```python
from build123d import *

# Parameters (mm, degrees)
F0_R     = 110
F0_R_2   = 1.75
F1_DEPTH = 3


with BuildPart() as f1:
    # F0 (on Top) → F1 (new body)
    with BuildSketch(Plane.XY):
        Circle(F0_R)
        with Locations((-91.582186, -52.875)):
            Circle(F0_R_2, mode=Mode.SUBTRACT)
        with Locations((0, -105.75)):
            Circle(F0_R_2, mode=Mode.SUBTRACT)
        with Locations((91.582186, -52.875)):
            Circle(F0_R_2, mode=Mode.SUBTRACT)
        with Locations((-91.582186, 52.875)):
            Circle(F0_R_2, mode=Mode.SUBTRACT)
        with Locations((91.582186, 52.875)):
            Circle(F0_R_2, mode=Mode.SUBTRACT)
        with Locations((0, 105.75)):
            Circle(F0_R_2, mode=Mode.SUBTRACT)
    extrude(amount=F1_DEPTH)


solid = f1.part
```
Here's how the part is built. I have some questions about the finished solid (model axes, mm). Give positions to 0.01 mm unless a question says otherwise; leave off trailing zeros. Loops run counter-clockwise (first coordinate to the right, second up) from the corner with the lowest first, then second, coordinate; pieces in that order, holes last. Notation, with made-up numbers: M 5.5,46 L 55.5,46 A17 cw 55.5,66 Z; hole C 25,-25.75 d1. An arc over 180 degrees is marked long. Use one line per item in the form item = value. Start each with the question number.
Q1. Thinking about a two-plate mould opening in Y: for faces 1 (the flat face through (-2, 2, 3)), 2 (the cylindrical face through (-23.846, -107.384, 1.479)), which applies, +Y half, -Y half, draft (parallel to the pull), parting line (faces both ways), or undercut?
Q2. Will these pins go through, and if not, where does the flat tip stop? pin 1 Ø1 at (y, z) = (-42.5, 2) entering from -X; pin 2 Ø5 at (x, y) = (-69, -82) entering from -Z; pin 3 Ø1.5 at (x, z) = (81, 2) entering from -Y.
Q3. If we section it at B-B (y = -73): Write out the boundary of the cut face in (x, z).
Q4. If we section it at A-A (z = 1.7): Write out the boundary of the cut face in (x, y) (3 decimals), then the cut area to 3 significant figures.
Q5. If we section it at C-C (x = -29.5): Write out the boundary of the cut face in (y, z).
Q6. I need wall thicknesses on line 1 along Y through (x, z) = (0, 1.9); line 2 along Y through (x, z) = (-90, 1.9); line 3 along Y through (x, z) = (14, 0.2). Which ranges of each line are inside material? Lowest first, please.
Taken from the geometry:
q1.face_1 = draft
q1.face_2 = parting line
q2.pin_1 = -101.67
q2.pin_2 = 0
q2.pin_3 = -75.23
q3.outline = M -82.29,0 L 82.29,0 L 82.29,3 L -82.29,3 Z
q4.outline = C 0,0 d220; hole C -91.582,-52.875 d3.5; hole C -91.582,52.875 d3.5; hole C 0,-105.75 d3.5; hole C 0,105.75 d3.5; hole C 91.582,-52.875 d3.5; hole C 91.582,52.875 d3.5
q4.area = 38,000 mm^2
q5.outline = M -105.97,0 L 105.97,0 L 105.97,3 L -105.97,3 Z
q6.line_1 = -110 to -107.5, -104 to 104, 107.5 to 110
q6.line_2 = -63.25 to -53.62, -52.13 to 52.13, 53.62 to 63.25
q6.line_3 = -109.11 to 109.11
